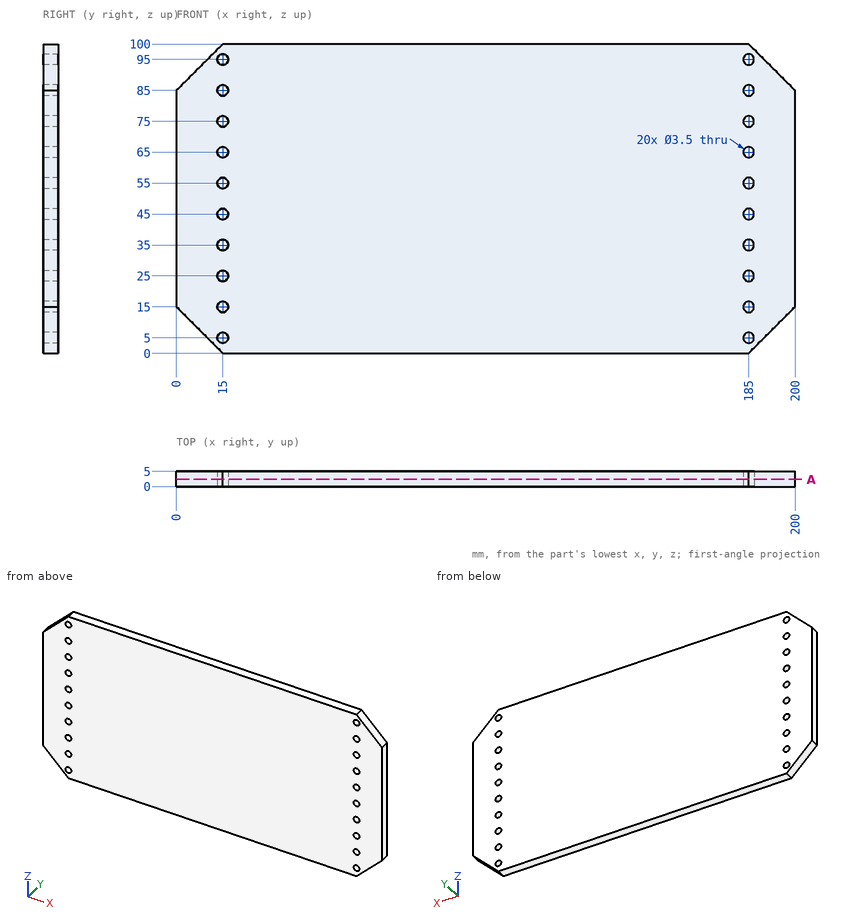
Geometry: see drawing. Coordinates: mm, zero at the bounding-box minimum. Round coordinates to 2 decimals unless told otherwise and drop trailing zeros. Write item = value, one per line. Start each with the question number.
(1) Pin query (flat end, axial travel): pin 1 (4.5 mm diameter, centred on x = 185, z = 15, fed in from +Y); pin 2 (2 mm diameter, centred on x = 15, z = 75, fed in from +Y). Return the tip coordinate at first contact, or that it passes through.
(2) Section query A-A, the plane y = 2.4. State how many separate pieces and enclosed holes the cut face has, plus the area to 3 significant figures.
(3) Ray query, line 1 along X through (y, z) = (1.2, 15); line 2 along X through (y, z) = (1.55, 44). Return the intervals inside material, ascending. Write a range as from..to.
Conclusion:
q1.pin_1 = 5
q1.pin_2 = through
q2.separate_pieces = 1
q2.enclosed_holes = 20
q2.area = 19,400 mm2
q3.line_1 = 0..13.25, 16.75..183.25, 186.75..200
q3.line_2 = 0..13.56, 16.44..183.56, 186.44..200
